Could you check a few things on this model? Use its own coordinates, in mm. A direction names the side the tool comes from. Give positions to 0.01 mm unless a question says otherwise; leave off trailing zeros. Order: outer loops, then holes, each group sorted by start corner. A loop starts at its lowest first (then second) coordinate and runs counter-clockwise, first axis right, second up. Notation, with made-up numbers: M 14,44 L 42,44 A14 cw 42,65 Z; hole C 46,3 d10. An arc over 180 degrees is marked long. Use a Markdown table: item, result. Add a question column.
Item 1: Suppose I cut it at B-B on z = 53.5. Write out the boundary of the cut face in (x, y) (3 decimals), plus the area to 3 significant figures.
Item 2: If I drill on L1, parallel to Y at x = 0, z = 1; L2, parallel to Y at x = -7.5, z = 17.5; L3, parallel to Z at x = -13, y = 6, over which ranges is the centre line in solid material (lowest first)? Write a range as from..to.
Item 3: For faces 4 (the face through (-7.606, 11, 31)), 5 (the face through (-11.693, -0.141, 30.853)), 6 (the face through (1.717, 0.541, 103.16)), 7 (the face through (7.123, -11.172, 2.12)), 8 (the face through (-7.606, -11, 31)), which set-ups out of +Z, -Z, +X, -X, +Y, -Y let a thin tool reach every point of the face, with its end or its side?
Item 4: Suppose I cut it at A-A on z = 105.5. Write out the boundary of the cut face in (x, y).
Item 5: I'm going to push flat-ended pins straight in: pin 1 Ø4 at (x, z) = (-0.5, 24) entering from +Y; pin 2 Ø6 at (x, y) = (-9.5, 6) entering from +Z; pin 3 Ø1 at (y, z) = (10, 36.5) entering from +X. Where does each tip first touch, or does it pass through?
Item 6: If we mould it in two halves opening along X, with no side actions, what happens to faces 1 (the face through (0, 0, 4.3)), 2 (the face through (-12, 0, 41.5)), 3 (the face through (14.435, 4.546, 32.955))? For each: released by +X, released by -X, zero draft, split by the parting line, or undercut.
from build123d import *

# Parameters (mm, degrees)
F0_R      = 14.5
F2_R      = 15.75
F4_R      = 13.25
F5_DEPTH  = 4.3
F8_DEPTH  = 21
F9_R      = 3.375
F10_DEPTH = 16
F11_R     = 0.5
F12_R     = 15.75
F13_DEPTH = 11
F17_R     = 1.8
F18_DEPTH = 25


with BuildPart() as f3:
    # F0 (on Top) → F3 section 0
    with BuildSketch(Plane.XY):
        Circle(F0_R)
    # F2 (on offset) → F3 section 1
    with BuildSketch(Plane.XY.offset(65)):
        Circle(F2_R)
    loft()

    # F4 (on face) → F5 (cut)
    with BuildSketch(Plane(origin=(0, 0, 0), x_dir=(1, 0, 0), z_dir=(0, 0, -1))):
        Circle(F4_R)
    extrude(amount=-F5_DEPTH, mode=Mode.SUBTRACT)

    # F7 (on offset) → F8 (cut)
    with BuildSketch(Plane.XY.offset(20.5)):
        with BuildLine():
            Line((-7.605769, -16.440997), (-7.605769, -12.805873))
            Line((-7.605769, -12.805873), (-7.605769, -8.882979))
            ThreePointArc((-7.605769, -8.882979), (-11.694231, 0), (-7.605769, 8.882979))
            Line((-7.605769, 8.882979), (-7.605769, 12.805873))
            Line((-7.605769, 12.805873), (-7.605769, 17.916933))
            Line((-7.605769, 17.916933), (-23.547225, 17.916933))
            Line((-23.547225, 17.916933), (-23.547225, -16.440997))
            Line((-23.547225, -16.440997), (-7.605769, -16.440997))
        make_face()
    extrude(amount=F8_DEPTH, mode=Mode.SUBTRACT)

    # F9 (on Front) → F10 (join)
    with BuildSketch(Plane.XZ):
        with Locations((0, 53.5)):
            Circle(F9_R)
    extrude(amount=F10_DEPTH)

    # F11
    f11_edges = [f3.edges().sort_by_distance(p)[0] for p in [
        (-3.375, -16, 53.5),
    ]]
    fillet(f11_edges, radius=F11_R)

    # F12 (on face) → F13 (join)
    with BuildSketch(Plane.XY.offset(65)):
        Circle(F12_R)
    extrude(amount=F13_DEPTH)

    # F14 (on Right) → F15 (revolve)
    with BuildSketch(Plane.YZ):
        with BuildLine():
            Line((0, 76), (15.75, 76))
            ThreePointArc((15.75, 76), (11.136932, 87.136932), (0, 91.75))
            Line((0, 91.75), (0, 76))
        make_face()
    revolve(axis=Axis((0, 0, 83.875), (0, 0, 1)))

    # F17 (on offset) → F18 (join)
    with BuildSketch(Plane.XY.offset(90)):
        Circle(F17_R)
    extrude(amount=F18_DEPTH)


solid = f3.part
Findings below:
| question | item | result |
|---|---|---|
| 1 | outline | M -3.375,-15.5 A0.5 ccw -2.875,-16 L 2.875,-16 A0.5 ccw 3.375,-15.5 L 3.375,-15.158 A15.529 ccw long -3.375,-15.158 Z |
| 1 | area | 761 mm^2 |
| 2 | L1 | y = -14.52..-13.25, 13.25..14.52 |
| 2 | L2 | y = -12.8..12.8 |
| 2 | L3 | z = 0..20.5, 41.5..82.56 |
| 3 | face 4 | -X, +Y |
| 3 | face 5 | -X |
| 3 | face 6 | +Z |
| 3 | face 7 | -Z |
| 3 | face 8 | -X, -Y |
| 4 | outline | C 0,0 d3.6 |
| 5 | pin 1 | stops at y = 15 |
| 5 | pin 2 | stops at z = 89.42 |
| 5 | pin 3 | stops at x = 11.87 |
| 6 | face 1 | undercut |
| 6 | face 2 | zero draft |
| 6 | face 3 | split by the parting line |
